Model file for the job. Use its own axes, mm. Face numbers are marked on the shaded views. A direction names the side the tool comes from. Coordinates: 2 decimals unless noted, no trailing zeros. Write each loop counter-clockwise with the first axis right and the second up, starting at its lowest first coordinate (ties: lowest second). Pieces come first, ordered by that corner, then holes. Notation, with made-up numbers: M 12.25,-27 L 67.25,-27 A3 cw 67.25,-22 Z; hole C 13,27 d5. An arc over 180 degrees is marked long. One line per question, with ' | ' between items. Start each with the question number.
(1) Flat gauge pins, fed straight in: pin 1 Ø4 at (x, y) = (23, 52) entering from +Z; pin 2 Ø6.5 at (x, y) = (-54.05, 22.39) entering from +Z. Where does each tip first touch, or does it go through?
(2) Tool access for the marked faces 5 and 6: list every direction of +Z, -Z, +X, -X, +Y, -Y with a clear straight run to the whole face (end or side of a thin tool).
(3) Wall check: probe 1 along Y at (x, z) = (-51, 3.5); probe 2 along Y at (x, z) = (-21, 8.75); probe 3 along Y at (x, z) = (1.5, 4.75). Give the ranges that are in metal, low to high.
(4) Cut at A-A (y = 0). Write the cut outline in (x, z).
(5) Cut at B-B (x = 0). Write the cut outline in (y, z), plus the area to 3 significant figures.
(6) Two-plate mould, pull along X, no slides. Class the marked faces 1, 2, 3 and 4: +X half, -X half, draft (parallel to the pull), parting line (faces both ways), or undercut.
(7) Cut at C-C (z = 5.5). Count the separate pieces of the cut face and the enclosed holes in it, plus the area to 3 significant figures.
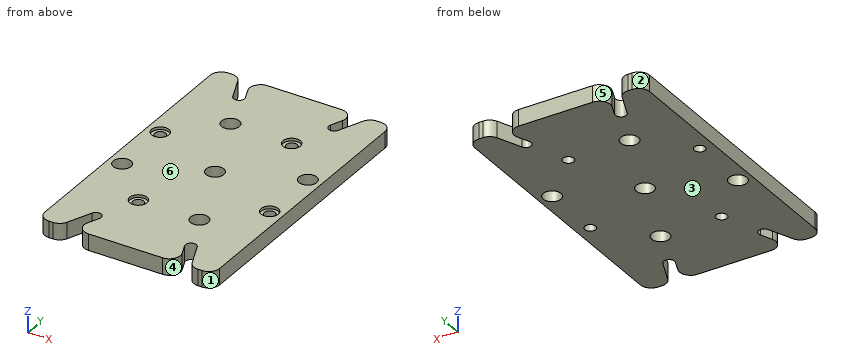
from build123d import *

# Parameters (mm, degrees)
F0_W      = 128
F0_H      = 210
F1_DEPTH  = 12
F2_R      = 8
F3_R      = 6.5
F3_R_2    = 4
F4_DEPTH  = 25
F3_R_3    = 6.35
F5_DEPTH  = 2
F7_DEPTH  = 25
F8_R      = 8
F10_R     = 6.5
F11_DEPTH = 25


with BuildPart() as f1:
    # F0 (on Top) → F1 (new body)
    with BuildSketch(Plane.XY):
        Rectangle(F0_W, F0_H)
    extrude(amount=F1_DEPTH)

    # F2
    f2_edges = [f1.edges().sort_by_distance(p)[0] for p in [
        (-64, -105, 6),
        (64, -105, 6),
        (64, 105, 6),
        (-64, 105, 6),
    ]]
    fillet(f2_edges, radius=F2_R)

    # F3 (on face) → F4 (cut)
    with BuildSketch(Plane.XY.offset(12)):
        with Locations((-22.3869807934, 54.0469526519)):
            Circle(F3_R)
        with Locations((-54.0469526519, 22.3869807934)):
            Circle(F3_R_2)
        with Locations((-54.0469526519, -22.3869807934)):
            Circle(F3_R)
        with Locations((-22.3869807934, -54.0469526519)):
            Circle(F3_R_2)
        with Locations((22.3869807934, -54.0469526519)):
            Circle(F3_R)
        with Locations((54.0469526519, -22.3869807934)):
            Circle(F3_R_2)
        with Locations((54.0469526519, 22.3869807934)):
            Circle(F3_R)
        with Locations((22.3869807934, 54.0469526519)):
            Circle(F3_R_2)
    extrude(amount=-F4_DEPTH, mode=Mode.SUBTRACT)

    # F3 (on face) → F5 (cut)
    with BuildSketch(Plane.XY.offset(12)):
        with Locations((-54.0469526519, 22.3869807934)):
            Circle(F3_R_3)
        with Locations((-54.0469526519, 22.3869807934)):
            Circle(F3_R_2, mode=Mode.SUBTRACT)
        with Locations((-22.3869807934, -54.0469526519)):
            Circle(F3_R_3)
        with Locations((-22.3869807934, -54.0469526519)):
            Circle(F3_R_2, mode=Mode.SUBTRACT)
        with Locations((54.0469526519, -22.3869807934)):
            Circle(F3_R_3)
        with Locations((54.0469526519, -22.3869807934)):
            Circle(F3_R_2, mode=Mode.SUBTRACT)
        with Locations((22.3869807934, 54.0469526519)):
            Circle(F3_R_3)
        with Locations((22.3869807934, 54.0469526519)):
            Circle(F3_R_2, mode=Mode.SUBTRACT)
    extrude(amount=-F5_DEPTH, mode=Mode.SUBTRACT)

    # F6 (on face) → F7 (cut)
    with BuildSketch(Plane.XY.offset(12)):
        with BuildLine():
            Line((-47.8209470608, 105), (-38.5524603376, 82.6238936502))
            Line((-38.5524603376, 82.6238936502), (-38.4851753385, 82.4614532928))
            ThreePointArc((-38.4851753385, 82.4614532928), (-33.2934586158, 80.3775193285), (-31.0959243529, 85.5221812669))
            Line((-31.0959243529, 85.5221812669), (-31.163209352, 85.6846216242))
            Line((-31.163209352, 85.6846216242), (-39.1639010376, 105))
            Line((-39.1639010376, 105), (-47.8209470608, 105))
        make_face()
        with BuildLine():
            Line((-38.5524603376, -82.6238936502), (-47.8209470608, -105))
            Line((-47.8209470608, -105), (-39.1639010376, -105))
            Line((-39.1639010376, -105), (-31.163209352, -85.6846216242))
            Line((-31.163209352, -85.6846216242), (-31.0959243529, -85.5221812669))
            ThreePointArc((-31.0959243529, -85.5221812669), (-33.2934586158, -80.3775193285), (-38.4851753385, -82.4614532928))
            Line((-38.4851753385, -82.4614532928), (-38.5524603376, -82.6238936502))
        make_face()
        with BuildLine():
            Line((31.163209352, -85.6846216242), (39.1639010376, -105))
            Line((39.1639010376, -105), (47.8209470608, -105))
            Line((47.8209470608, -105), (38.5524603376, -82.6238936502))
            Line((38.5524603376, -82.6238936502), (38.4851753385, -82.4614532928))
            ThreePointArc((38.4851753385, -82.4614532928), (33.2934586158, -80.3775193285), (31.0959243529, -85.5221812669))
            Line((31.0959243529, -85.5221812669), (31.163209352, -85.6846216242))
        make_face()
        with BuildLine():
            Line((47.8209470608, 105), (39.1639010376, 105))
            Line((39.1639010376, 105), (31.163209352, 85.6846216242))
            Line((31.163209352, 85.6846216242), (31.0959243529, 85.5221812669))
            ThreePointArc((31.0959243529, 85.5221812669), (33.2934586158, 80.3775193285), (38.4851753385, 82.4614532928))
            Line((38.4851753385, 82.4614532928), (38.5524603376, 82.6238936502))
            Line((38.5524603376, 82.6238936502), (47.8209470608, 105))
        make_face()
    extrude(amount=-F7_DEPTH, mode=Mode.SUBTRACT)

    # F8
    f8_edges = [f1.edges().sort_by_distance(p)[0] for p in [
        (-47.820947, 105, 6),
        (-39.163901, 105, 6),
        (39.163901, 105, 6),
        (47.820947, 105, 6),
        (47.820947, -105, 6),
        (39.163901, -105, 6),
        (-39.163901, -105, 6),
        (-47.820947, -105, 6),
    ]]
    fillet(f8_edges, radius=F8_R)

    # F10 (on face) → F11 (cut)
    with BuildSketch(Plane.XY.offset(12)):
        Circle(F10_R)
    extrude(amount=-F11_DEPTH, mode=Mode.SUBTRACT)


solid = f1.part
Filled in:
1) pin 1: z = 10 | pin 2: through
2) face 5: +Z, -Z | face 6: +Z, +X, -X, +Y, -Y
3) probe 1: -104.7 to -28.13, -16.65 to 19.8, 24.98 to 104.7 | probe 2: -105 to -57.8, -50.3 to 47.7, 60.4 to 105 | probe 3: -105 to -6.32, 6.32 to 105
4) outline: M -64,0 L -6.5,0 L -6.5,12 L -64,12 Z; M 6.5,0 L 64,0 L 64,12 L 6.5,12 Z
5) outline: M -105,0 L -6.5,0 L -6.5,12 L -105,12 Z; M 6.5,0 L 105,0 L 105,12 L 6.5,12 Z | area: 2,360 mm²
6) face 1: +X half | face 2: -X half | face 3: draft | face 4: undercut
7) separate pieces: 1 | enclosed holes: 9 | area: 25,000 mm²
